Model file for the job. Use its own axes, mm. A direction names the side the tool comes from. Give positions to 0.01 mm unless a question says otherwise; leave off trailing zeros. Loops run counter-clockwise (first coordinate to the right, second up) from the corner with the lowest first, then second, coordinate; pieces in that order, holes last. Notation, with made-up numbers: (72.5, 50.25) - (101.5, 50.25) arc R34 ccw to (101.5, 80.25) - close; hole circle Ø4 at (28, -22). An arc over 180 degrees is marked (long way). Answer as CSV lines item,"result". Start each with the question number.
Item 1: Saw through at A-A on x = 34. Give the cut face in (y, z) (3 decimals), plus the area to 3 significant figures.
Item 2: Saw through at D-D on z = -18.8. Give the cut face in (x, y), plus the area to 3 significant figures.
Item 3: Drill centre lines: L1, parallel to X at y = 0.95, z = -12.5 (3 decimals); L2, parallel to X at y = 1.75, z = -5.75; L3, parallel to X at y = 0.7, z = -5.5. Where is each one in solid material? Low to high. Write a range as from..to.
Item 4: Saw through at C-C on y = 0.6. Give the cut face in (x, z) (3 decimals), plus the area to 3 significant figures.
Item 5: Saw through at B-B on z = -12.5. Give the cut face in (x, y) (3 decimals), plus the area to 4 significant figures.
Item 6: Tool access for faces 5 (the flat face through (2, 1, -10.425)), 6 (the flat face through (19, 1, 0)): list every direction of +Z, -Z, +X, -X, +Y, -Y with a clear straight run to the whole face (end or side of a thin tool).
Item 7: Pull direction Z, two halves, no side cores. Call faces 1 (the cylindrical face through (37, 1, -6.2)), 2 (the flat face through (19, 0, -13)), 3 (the cylindrical face through (1, 1, -6.2)), 4 (the flat face through (37, 1, -24)): pulls with the +Z half, pulls with the -Z half, needs draft (parallel to the pull), parting line crosses it, or undercut.
from build123d import *

# Parameters (mm, degrees)
SKETCH1_R      = 2.075
EXTRUDE1_DEPTH = 2


with BuildPart() as part:
    # Sketch1 → Extrude1 (new body)
    with BuildSketch(Plane(origin=(0, 0, 0), x_dir=(1, 0, 0), z_dir=(0, 1, 0))):
        with BuildLine():
            Line((2, 0), (36, 0))
            Line((36, 0), (38, 2))
            Line((38, 2), (38, 5.2))
            ThreePointArc((38, 5.2), (37, 6.2), (38, 7.2))
            Line((38, 7.2), (38, 17.8))
            ThreePointArc((38, 17.8), (37, 18.8), (38, 19.8))
            Line((38, 19.8), (38, 23))
            Line((38, 23), (36, 25))
            Line((36, 25), (2, 25))
            Line((2, 25), (0, 23))
            Line((0, 23), (0, 19.8))
            ThreePointArc((0, 19.8), (1, 18.8), (0, 17.8))
            Line((0, 17.8), (0, 14.575))
            Line((0, 14.575), (4, 14.575))
            ThreePointArc((4, 14.575), (6.075, 12.5), (4, 10.425))
            Line((4, 10.425), (0, 10.425))
            Line((0, 10.425), (0, 7.2))
            ThreePointArc((0, 7.2), (1, 6.2), (0, 5.2))
            Line((0, 5.2), (0, 2))
            Line((0, 2), (2, 0))
        make_face()
        with Locations(Location((34, 12.5, 0), (0, 0, 270))):  # turned: the seam where the file's is
            Circle(SKETCH1_R, mode=Mode.SUBTRACT)
    extrude(amount=EXTRUDE1_DEPTH)


solid = part.part
Responses:
1,outline,"(0, -25) - (2, -25) - (2, -14.575) - (0, -14.575) - close; (0, -10.425) - (2, -10.425) - (2, 0) - (0, 0) - close"
1,area,"41.7 mm2"
2,outline,"(1, 0) - (37, 0) - (37, 2) - (1, 2) - close"
2,area,"72.0 mm2"
3,L1,"6.075..31.925, 36.075..38"
3,L2,"0.89..37.11"
3,L3,"0.71..37.29"
4,outline,"(0, -23) - (2, -25) - (36, -25) - (38, -23) - (38, -19.8) arc R1 cw to (38, -17.8) - (38, -7.2) arc R1 cw to (38, -5.2) - (38, -2) - (36, 0) - (2, 0) - (0, -2) - (0, -5.2) arc R1 cw to (0, -7.2) - (0, -10.425) - (4, -10.425) arc R2.075 cw to (4, -14.575) - (0, -14.575) - (0, -17.8) arc R1 cw to (0, -19.8) - close; hole circle Ø4.15 at (34, -12.5)"
4,area,"899 mm2"
5,outline,"(6.075, 0) - (31.925, 0) - (31.925, 2) - (6.075, 2) - close; (36.075, 0) - (38, 0) - (38, 2) - (36.075, 2) - close"
5,area,"55.55 mm2"
6,face 5,"-X, +Y, -Y"
6,face 6,"+Z, +X, -X, +Y, -Y"
7,face 1,"undercut"
7,face 2,"needs draft"
7,face 3,"undercut"
7,face 4,"pulls with the -Z half"
